from build123d import *

# Parameters (mm, degrees)
BOSS_EXTRUDE5_DEPTH = 84.074
SKETCH12_R          = 2.38125
BOSS_EXTRUDE6_DEPTH = 3.175


with BuildPart() as part:
    # Sketch11 → Boss-Extrude5 (new body)
    with BuildSketch(Plane(origin=(0, 0, 0), x_dir=(0, 0, -1), z_dir=(1, 0, 0))):
        with BuildLine():
            Line((0, 2.54), (0, 85.979))
            ThreePointArc((0, 85.979), (-0.371974388, 86.877025612), (-1.27, 87.249))
            Line((-1.27, 87.249), (-1.905, 87.249))
            ThreePointArc((-1.905, 87.249), (-2.803025612, 86.877025612), (-3.175, 85.979))
            Line((-3.175, 85.979), (-3.175, 3.175))
            Line((-3.175, 3.175), (-83.947, 3.175))
            ThreePointArc((-83.947, 3.175), (-84.845025612, 2.803025612), (-85.217, 1.905))
            Line((-85.217, 1.905), (-85.217, 1.27))
            ThreePointArc((-85.217, 1.27), (-84.845025612, 0.371974388), (-83.947, 0))
            Line((-83.947, 0), (-2.54, 0))
            ThreePointArc((-2.54, 0), (-0.743948776, 0.743948776), (0, 2.54))
        make_face()
    extrude(amount=BOSS_EXTRUDE5_DEPTH)

    # Sketch12 → Boss-Extrude6 (add)
    with BuildSketch(Plane(origin=(84.074, 0, 0), x_dir=(0, 0, -1), z_dir=(1, 0, 0))):
        with BuildLine():
            Line((-49.75225, -18.328132), (-49.75225, 0))
            Line((-49.75225, 0), (-35.46475, 0))
            Line((-35.46475, 0), (-35.46475, -18.328132))
            ThreePointArc((-35.46475, -18.328132), (-35.836724388, -19.226157612), (-36.73475, -19.598132))
            Line((-36.73475, -19.598132), (-48.48225, -19.598132))
            ThreePointArc((-48.48225, -19.598132), (-49.380275612, -19.226157612), (-49.75225, -18.328132))
        make_face()
        with Locations((-42.6085, -12.454382)):
            Circle(SKETCH12_R, mode=Mode.SUBTRACT)
    extrude(amount=-BOSS_EXTRUDE6_DEPTH)


solid = part.part
Input: part model. Units: mm. Frame: model coordinates. A direction names the side the tool comes from. Give positions to 0.01 mm unless a question says otherwise; leave off trailing zeros. Loops run counter-clockwise (first coordinate to the right, second up) from the corner with the lowest first, then second, coordinate; pieces in that order, holes last. Notation, with made-up numbers: (-11.5, 70) -> (-2.5, 70) arc R30 ccw to (-2.5, 94) -> close; hole circle Ø8 at (-32.75, 40.25). An arc over 180 degrees is marked (long way). Answer as a JSON object with one key per item and string values. Group by question number.
Item 1: Cut plane C-C, the plane y = 74.5. Return the cut outline in (x, z) (3 decimals), and give its area (3 significant figures).
Item 2: Pin query (flat end, axial travel): P1, Ø7.5, axis at y = -12.45, z = 42.61, coming from the -X side; P2, Ø4, axis at x = 26, z = 26, coming from the -Y side; P3, Ø25, axis at x = 62.5, y = 62.5, coming from the +Z side (3 decimals). Return the tip coordinate at first contact, or that it passes through.
Item 3: Reachability of faces 4 (the flat face through (41, 3.175, 43)), 5 (the flat face through (80.899, -9.7, 42.5)), 6 (the flat face through (83, -9, 35.465)) from +Z, -Z, +X, -X, +Y, -Y: full face, straight path, thin tool, end or side. Return the list, or none.
Item 4: Cut plane B-B, the plane x = 62. Return the cut outline in (y, z) (3 decimals), and give its area (3 significant figures).
Item 5: Line query: probe 1 along Z at (x, y) = (61.5, 26.5) (3 decimals). Output: solid intervals per line, ascending.
Item 6: Cut plane A-A, the plane z = 42. Return the cut outline in (x, y) (3 decimals), and give its area (3 significant figures).
Item 7: Pull-direction query (Z, two-part tool) for faces 1 (the flat face through (84.074, 2, 30)), 2 (the flat face through (41, 45, 3.175)), 3 (the cylindrical face through (82.5, -13.9, 44.5)); classes: released by +Z, released by -Z, zero draft, split by the parting line, or undercut.
Checks:
{
 "1": {"outline": "(0, 0) -> (84.074, 0) -> (84.074, 3.175) -> (0, 3.175) -> close", "area": "267 mm²"},
 "2": {"P1": "stops at x = 80.9", "P2": "stops at y = 0", "P3": "stops at z = 3.175"},
 "3": {"face 4": "+Z, +X, -X, +Y", "face 5": "+Z, -Z, -X, -Y", "face 6": "-Z, +X, -X, -Y"},
 "4": {"outline": "(0, 2.54) arc R2.54 ccw to (2.54, 0) -> (85.979, 0) arc R1.27 ccw to (87.249, 1.27) -> (87.249, 1.905) arc R1.27 ccw to (85.979, 3.175) -> (3.175, 3.175) -> (3.175, 83.947) arc R1.27 ccw to (1.905, 85.217) -> (1.27, 85.217) arc R1.27 ccw to (0, 83.947) -> close", "area": "535 mm²"},
 "5": {"probe 1": "z = 0 to 3.175"},
 "6": {"outline": "(0, 0) -> (80.899, 0) -> (80.899, -10.152) -> (84.074, -10.152) -> (84.074, 3.175) -> (0, 3.175) -> close; (80.899, -19.598) -> (84.074, -19.598) -> (84.074, -14.757) -> (80.899, -14.757) -> close", "area": "315 mm²"},
 "7": {"face 1": "zero draft", "face 2": "released by +Z", "face 3": "undercut"}
}
